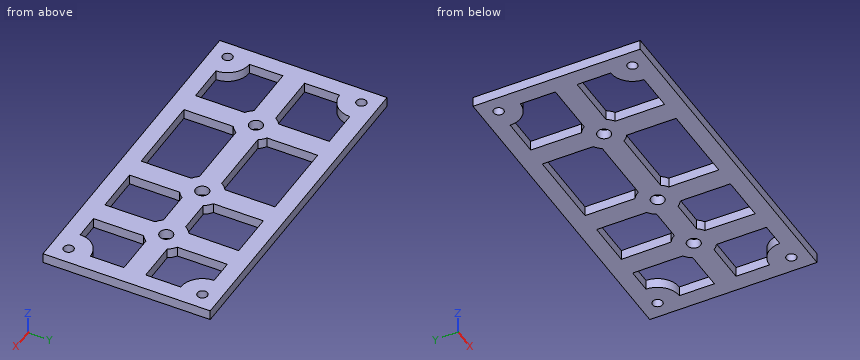
```python
from build123d import *

# Parameters (mm, degrees)
SKETCH1_W               = 115
SKETCH1_H               = 50
BOSS_EXTRUDE1_DEPTH     = 3
CUT_EXTRUDE1_START      = -4
SKETCH2_R               = 1.5
CUT_EXTRUDE1_DEPTH      = 5
SKETCH4_R               = 2
CUT_EXTRUDE2_DEPTH      = 4
SKETCH5_R               = 2
CUT_EXTRUDE3_DEPTH      = 10
SKETCH6_R               = 2
CUT_EXTRUDE4_DEPTH      = 10
SKETCH7_W               = 15.674157042
SKETCH7_H               = 50
CUT_EXTRUDE5_DEPTH      = 10
MIRROR2_START           = -4
MIRROR2_COPY_1_SKETCH_R = 1.5
MIRROR2_COPY_1_DEPTH    = 5
CUT_EXTRUDE6_DEPTH      = 10


with BuildPart() as part:
    # Sketch1 → Boss-Extrude1 (new body)
    with BuildSketch(Plane.XY):
        Rectangle(SKETCH1_W, SKETCH1_H)
    extrude(amount=BOSS_EXTRUDE1_DEPTH)

    # Sketch2 → Cut-Extrude1 (cut)
    with BuildSketch(Plane.XY.offset(3).offset(CUT_EXTRUDE1_START)):
        with Locations((-52.5, 20)):
            Circle(SKETCH2_R)
    cut_extrude1 = extrude(amount=CUT_EXTRUDE1_DEPTH, mode=Mode.SUBTRACT)

    # Sketch4 → Cut-Extrude2 (cut, through all)
    with BuildSketch(Plane.XY.offset(3)):
        with Locations((-31.210457155, -0.20944607)):
            Circle(SKETCH4_R)
    extrude(amount=-CUT_EXTRUDE2_DEPTH, mode=Mode.SUBTRACT)

    # Sketch5 → Cut-Extrude3 (cut)
    with BuildSketch(Plane.XY.offset(3)):
        with Locations((-0.691956257, 0)):
            Circle(SKETCH5_R)
    extrude(amount=-CUT_EXTRUDE3_DEPTH, mode=Mode.SUBTRACT)

    # Sketch6 → Cut-Extrude4 (cut)
    with BuildSketch(Plane.XY.offset(3)):
        with Locations((19.565842958, 0)):
            Circle(SKETCH6_R)
    extrude(amount=-CUT_EXTRUDE4_DEPTH, mode=Mode.SUBTRACT)

    # Sketch7 → Cut-Extrude5 (cut)
    with BuildSketch(Plane.XY.offset(3)):
        with Locations((49.662921479, 0)):
            Rectangle(SKETCH7_W, SKETCH7_H)
    extrude(amount=-CUT_EXTRUDE5_DEPTH, mode=Mode.SUBTRACT)

    # Mirror1: Cut-Extrude1 across plane
    add(cut_extrude1.mirror(Plane.ZY.offset(7.837078521)), mode=Mode.SUBTRACT)

    # Mirror2: Cut-Extrude1 across plane
    add(cut_extrude1.mirror(Plane.ZX), mode=Mode.SUBTRACT)

    # Mirror2 copy 1 sketch → Mirror2 copy 1 (cut)
    with BuildSketch(Plane(origin=(-15.674157042, 0, 3), x_dir=(-1, 0, 0), z_dir=(0, 0, 1)).offset(MIRROR2_START)):
        with Locations((-52.5, 20)):
            Circle(MIRROR2_COPY_1_SKETCH_R)
    extrude(amount=MIRROR2_COPY_1_DEPTH, mode=Mode.SUBTRACT)

    # Sketch8 → Cut-Extrude6 (cut)
    with BuildSketch(Plane.XY.offset(3)):
        with BuildLine():
            ThreePointArc((-52.5, 13.5), (-47.903805922, 15.403805922), (-46, 20))
            Line((-46, 20), (-34.460457155, 20))
            Line((-34.460457155, 20), (-34.460457155, 4.834114181))
            ThreePointArc((-34.460457155, 4.834114181), (-35.453097842, 4.033194618), (-36.254017405, 3.04055393))
            Line((-36.254017405, 3.04055393), (-52.5, 3.04055393))
            Line((-52.5, 3.04055393), (-52.5, 13.5))
        make_face()
        with BuildLine():
            ThreePointArc((-3.941956257, 5.04356025), (-5.020668226, 4.15478672), (-5.864482893, 3.04055393))
            Line((-5.864482893, 3.04055393), (-26.166896904, 3.04055393))
            ThreePointArc((-26.166896904, 3.04055393), (-26.967816468, 4.033194618), (-27.960457155, 4.834114181))
            Line((-27.960457155, 4.834114181), (-27.960457155, 20))
            Line((-27.960457155, 20), (-3.941956257, 20))
            Line((-3.941956257, 20), (-3.941956257, 5.04356025))
        make_face()
        with BuildLine():
            ThreePointArc((4.480570379, 3.04055393), (3.636755712, 4.15478672), (2.558043743, 5.04356025))
            Line((2.558043743, 5.04356025), (2.558043743, 20))
            Line((2.558043743, 20), (16.44194335, 20))
            Line((16.44194335, 20), (16.347771528, 5.063992128))
            ThreePointArc((16.347771528, 5.063992128), (15.250277003, 4.168439815), (14.393316322, 3.04055393))
            Line((14.393316322, 3.04055393), (4.480570379, 3.04055393))
        make_face()
        with BuildLine():
            Line((36.825842958, 3.04055393), (36.825842958, 13.5))
            ThreePointArc((36.825842958, 13.5), (32.22964888, 15.403805922), (30.325842958, 20))
            Line((30.325842958, 20), (22.815842958, 20))
            Line((22.815842958, 20), (22.815842958, 5.04356025))
            ThreePointArc((22.815842958, 5.04356025), (23.894554927, 4.15478672), (24.738369593, 3.04055393))
            Line((24.738369593, 3.04055393), (36.825842958, 3.04055393))
        make_face()
        with BuildLine():
            Line((36.825842958, -13.5), (36.825842958, -3.45944607))
            Line((36.825842958, -3.45944607), (24.468111095, -3.45944607))
            ThreePointArc((24.468111095, -3.45944607), (23.718218589, -4.331024892), (22.815842958, -5.04356025))
            Line((22.815842958, -5.04356025), (22.815842958, -20))
            Line((22.815842958, -20), (30.325842958, -20))
            ThreePointArc((30.325842958, -20), (32.22964888, -15.403805922), (36.825842958, -13.5))
        make_face()
        with BuildLine():
            ThreePointArc((14.66357482, -3.45944607), (15.427169174, -4.344120085), (16.347771528, -5.063992128))
            Line((16.347771528, -5.063992128), (16.44194335, -20))
            Line((16.44194335, -20), (2.558043743, -20))
            Line((2.558043743, -20), (2.558043743, -5.04356025))
            ThreePointArc((2.558043743, -5.04356025), (3.460419374, -4.331024892), (4.21031188, -3.45944607))
            Line((4.21031188, -3.45944607), (14.66357482, -3.45944607))
        make_face()
        with BuildLine():
            ThreePointArc((-27.960457155, -5.25300632), (-26.967816468, -4.452086757), (-26.166896904, -3.45944607))
            Line((-26.166896904, -3.45944607), (-5.594224394, -3.45944607))
            ThreePointArc((-5.594224394, -3.45944607), (-4.844331888, -4.331024892), (-3.941956257, -5.04356025))
            Line((-3.941956257, -5.04356025), (-3.941956257, -20))
            Line((-3.941956257, -20), (-27.960457155, -20))
            Line((-27.960457155, -20), (-27.960457155, -5.25300632))
        make_face()
        with BuildLine():
            ThreePointArc((-36.254017405, -3.45944607), (-35.453097842, -4.452086757), (-34.460457155, -5.25300632))
            Line((-34.460457155, -5.25300632), (-34.460457155, -20))
            Line((-34.460457155, -20), (-46, -20))
            ThreePointArc((-46, -20), (-47.903805922, -15.403805922), (-52.5, -13.5))
            Line((-52.5, -13.5), (-52.5, -3.45944607))
            Line((-52.5, -3.45944607), (-36.254017405, -3.45944607))
        make_face()
    extrude(amount=-CUT_EXTRUDE6_DEPTH, mode=Mode.SUBTRACT)


solid = part.part
```
Can you work these out from the model? Positions are in its coordinate system, mm. Round coordinates to 2 decimals unless told otherwise and drop trailing zeros. Loops run counter-clockwise (first coordinate to the right, second up) from the corner with the lowest first, then second, coordinate; pieces in that order, holes last. Notation, with made-up numbers: (71.5, 64) -> (120.5, 64) arc R37 ccw to (120.5, 101) -> close; hole circle Ø10 at (-4, 9). An arc over 180 degrees is marked (long way). One line per item, written item: value. Start each with the question number.
1. If we section it at C-C, the plane x = 0: Write out the boundary of the cut face in (y, z).
2. If we section it at D-D, the plane z = 1.75: Give the number of separate pieces and of enclosed holes in the cut face, then the cut area to 3 significant figures.
3. For pin 1 (2.5 mm diameter, centred on x = 36.83, y = 20, fed in from +Z), with a flat end and sliding along its axis, tell me the tip position at first contact or that it passes through.
4. If I drill on probe 1 along X at (y, z) = (6, 2.3); probe 2 along Y at (x, z) = (-42.5, 1.9); probe 3 along Y at (x, z) = (-35, 1.05), over which ranges is the centre line in solid material (lowest first)?
5. If we section it at B-B, the plane y = -15: Write out the boundary of the cut face in (x, z).
6. If we section it at A-A, the plane x = 11.5: Write out the boundary of the cut face in (y, z), then the cut area to 3 significant figures.
Calculated:
1. outline: (-25, 0) -> (-1.88, 0) -> (-1.88, 3) -> (-25, 3) -> close; (1.88, 0) -> (25, 0) -> (25, 3) -> (1.88, 3) -> close
2. separate pieces: 1
2. enclosed holes: 15
2. area: 2,710 mm²
3. pin 1: passes through
4. probe 1: x = -57.5 to -52.5, -34.46 to -27.96, -3.94 to 2.56, 16.35 to 22.82, 36.83 to 41.83
4. probe 2: y = -25 to -20, -3.46 to 3.04, 20 to 25
4. probe 3: y = -25 to -20, -4.86 to 4.44, 20 to 25
5. outline: (-57.5, 0) -> (-48.35, 0) -> (-48.35, 3) -> (-57.5, 3) -> close; (-34.46, 0) -> (-27.96, 0) -> (-27.96, 3) -> (-34.46, 3) -> close; (-3.94, 0) -> (2.56, 0) -> (2.56, 3) -> (-3.94, 3) -> close; (16.41, 0) -> (22.82, 0) -> (22.82, 3) -> (16.41, 3) -> close; (32.67, 0) -> (41.83, 0) -> (41.83, 3) -> (32.67, 3) -> close
6. outline: (-25, 0) -> (-20, 0) -> (-20, 3) -> (-25, 3) -> close; (-3.46, 0) -> (3.04, 0) -> (3.04, 3) -> (-3.46, 3) -> close; (20, 0) -> (25, 0) -> (25, 3) -> (20, 3) -> close
6. area: 49.5 mm²
